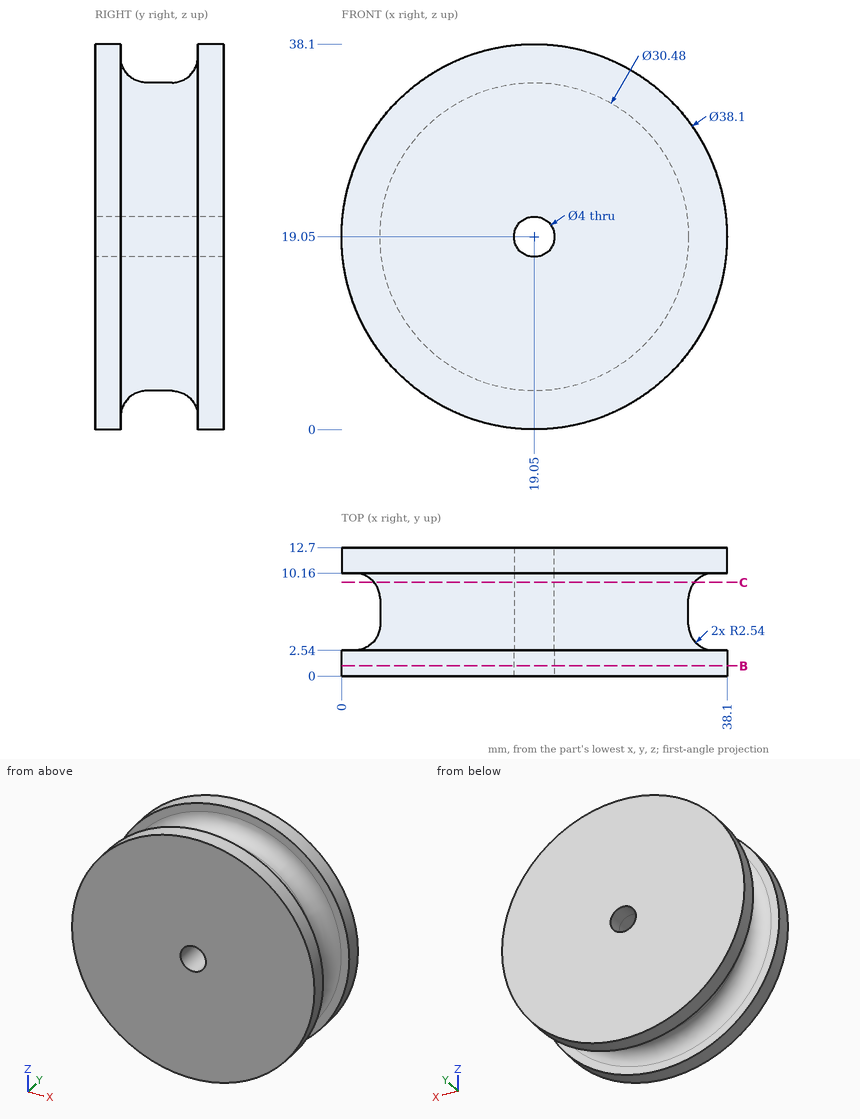
Design review of the part shown in the three views and the two pictorial views. Dimensions are in mm from the part's minimum x, y and z. Give positions to 0.01 mm unless a question says otherwise; leave off trailing zeros. Loops run counter-clockwise (first coordinate to the right, second up) from the corner with the lowest first, then second, coordinate; pieces in that order, holes last. Notation, with made-up numbers: M 59,-3 L 65,-3 A33 cw 65,31 Z; hole C 64.25,58.25 d11. An arc over 180 degrees is marked long. Answer as a JSON object with one key per item and string values.
Item 1: Wall thickness on line 1 along Z through (x, y) = (19.05, 12.1); line 2 along Y through (x, z) = (30, 4): over which ranges is each line inside the solid? List them lowest first.
Output values:
{"line 1": "z = 0 to 17.05, 21.05 to 38.1", "line 2": "y = 0 to 2.54, 10.16 to 12.7"}
Item 2: For P1, Ø5, axis at x = 4.5, z = 26, coming from the -Y side; P2, Ø5, axis at x = 10, y = 2, coming from the -Z side; P3, Ø3.5, axis at x = 19.05, z = 19.05, coming from the +Y side; P4, Ø1.5, axis at y = 6.5, z = 8, coming from the -X side, all flat-tipped, find the tip position at first contact; note any pin that passes through.
Output values:
{"P1": "stops at y = 0", "P2": "stops at z = 1.16", "P3": "passes through", "P4": "stops at x = 7.82"}
Item 3: We need section B-B (y = 1). State the section outline as (x, z) points, and give its area (3 significant figures).
Output values:
{"outline": "C 19.05,19.05 d38.1; hole C 19.05,19.05 d4", "area": "1,130 mm2"}
Item 4: We need section C-C (y = 9.25). State the section outline as (x, z) points, and give its area (3 significant figures).
Output values:
{"outline": "C 19.05,19.05 d31.66; hole C 19.05,19.05 d4", "area": "775 mm2"}
